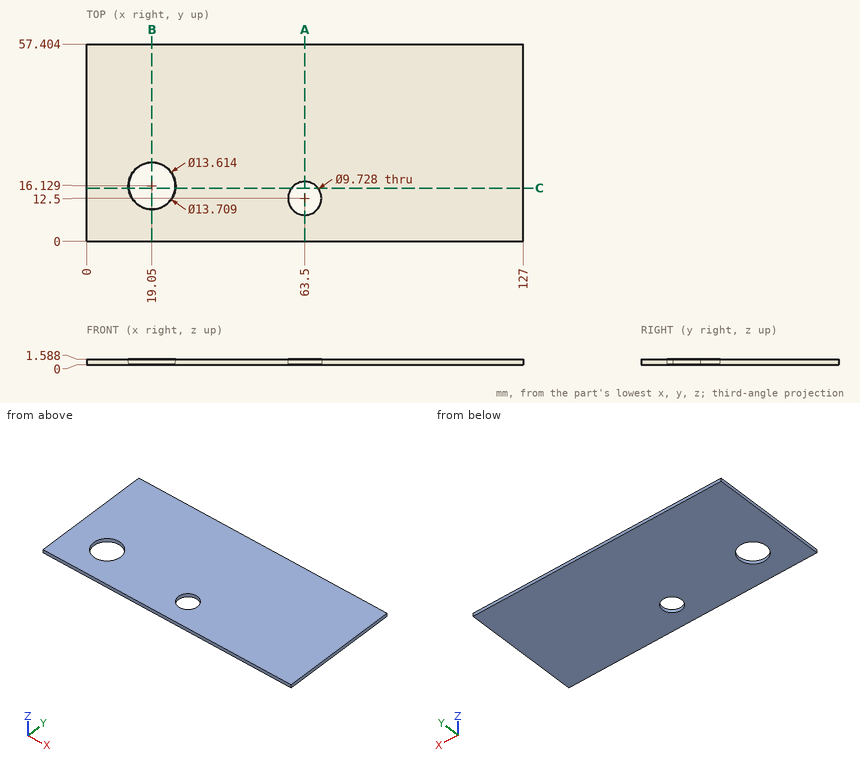
Print and shaded views of the part. All mm, measured from the part's lowest x, y and z. Give positions to 0.01 mm unless a question says otherwise; leave off trailing zeros. Loops run counter-clockwise (first coordinate to the right, second up) from the corner with the lowest first, then second, coordinate; pieces in that order, holes last.
1) Saw through at A-A (x = 63.5). Write the cut outline in (y, z) (1 decimal).
2) Wall check: line 1 (Y direction, x = 63.5, z = 0.85) (1 decimal); line 2 (X direction, y = 10.5, z = 0.35) (1 decimal); line 3 (X direction, y = 21.5, z = 0.25) (1 decimal). Give the ranges that are in metal, low to high.
3) Saw through at B-B (x = 19.05). Write the cut outline in (y, z) (1 decimal).
4) Saw through at C-C (y = 15.5). Count the separate pieces of the cut face and the enclosed holes in it, plus the area to 3 significant figures.
Answer block:
1. outline: (0, 0) - (7.6, 0) - (7.6, 1.6) - (0, 1.6) - close; (17.4, 0) - (57.4, 0) - (57.4, 1.6) - (17.4, 1.6) - close
2. line 1: y = 0 to 7.6, 17.4 to 57.4
2. line 2: x = 0 to 15.2, 22.9 to 59.1, 67.9 to 127
2. line 3: x = 0 to 14.9, 23.2 to 127
3. outline: (0, 0) - (9.3, 0) - (9.3, 1.6) - (0, 1.6) - close; (22.9, 0) - (57.4, 0) - (57.4, 1.6) - (23, 1.6) - close
4. separate pieces: 3
4. enclosed holes: 0
4. area: 168 mm2
